```python
from build123d import *

# Parameters (mm, degrees)
SWEEP_THIN1_PROFILE_R   = 15
SWEEP_THIN1_PROFILE_R_2 = 11
SKETCH65_R              = 11
SKETCH65_R_2            = 3
BOSS_EXTRUDE1_DEPTH     = 5
SKETCH66_R              = 11
SKETCH66_R_2            = 3
BOSS_EXTRUDE2_DEPTH     = 5


with BuildPart() as part:
    # Sweep-Thin1: sweep along a path in Sketch1
    with BuildLine(Plane.XY) as sweep_thin1_path:
        ThreePointArc((-45, 0), (-31.819805153, 31.819805153), (0, 45))
    # Sweep-Thin1 profile (on start of the path) → Sweep-Thin1 (sweep)
    with BuildSketch(Plane(origin=(-45, 0, 0), x_dir=(1, 0, 0), z_dir=(0, 1, 0))):
        Circle(SWEEP_THIN1_PROFILE_R)
        Circle(SWEEP_THIN1_PROFILE_R_2, mode=Mode.SUBTRACT)
    sweep(path=sweep_thin1_path.line)

    # Sketch65 → Boss-Extrude1 (add)
    with BuildSketch(Plane(origin=(0, 0, 0), x_dir=(0, 0, -1), z_dir=(1, 0, 0))):
        with BuildLine():
            Line((-5.157087895, 70.566666667), (-15.04150636, 53.944444444))
            ThreePointArc((-15.04150636, 53.944444444), (-17.5, 45), (-15.04150636, 36.055555556))
            Line((-15.04150636, 36.055555556), (-5.157087895, 19.433333333))
            ThreePointArc((-5.157087895, 19.433333333), (0, 16.5), (5.157087895, 19.433333333))
            Line((5.157087895, 19.433333333), (15.04150636, 36.055555556))
            ThreePointArc((15.04150636, 36.055555556), (17.5, 45), (15.04150636, 53.944444444))
            Line((15.04150636, 53.944444444), (5.157087895, 70.566666667))
            ThreePointArc((5.157087895, 70.566666667), (0, 73.5), (-5.157087895, 70.566666667))
        make_face()
        with Locations(Location((0, 45, 0), (0, 0, 90))):
            Circle(SKETCH65_R, mode=Mode.SUBTRACT)
        with Locations(Location((0, 67.5, 0), (0, 0, 90))):
            Circle(SKETCH65_R_2, mode=Mode.SUBTRACT)
        with Locations(Location((0, 22.5, 0), (0, 0, 90))):
            Circle(SKETCH65_R_2, mode=Mode.SUBTRACT)
    extrude(amount=BOSS_EXTRUDE1_DEPTH)

    # Sketch66 → Boss-Extrude2 (add)
    with BuildSketch(Plane.XZ):
        with BuildLine():
            Line((-53.944444444, 15.04150636), (-70.566666667, 5.157087895))
            ThreePointArc((-70.566666667, 5.157087895), (-73.5, 0), (-70.566666667, -5.157087895))
            Line((-70.566666667, -5.157087895), (-53.944444444, -15.04150636))
            ThreePointArc((-53.944444444, -15.04150636), (-45, -17.5), (-36.055555556, -15.04150636))
            Line((-36.055555556, -15.04150636), (-19.433333333, -5.157087895))
            ThreePointArc((-19.433333333, -5.157087895), (-16.5, 0), (-19.433333333, 5.157087895))
            Line((-19.433333333, 5.157087895), (-36.055555556, 15.04150636))
            ThreePointArc((-36.055555556, 15.04150636), (-45, 17.5), (-53.944444444, 15.04150636))
        make_face()
        with Locations(Location((-45, 0, 0), (0, 0, 180))):
            Circle(SKETCH66_R, mode=Mode.SUBTRACT)
        with Locations((-67.5, 0)):
            Circle(SKETCH66_R_2, mode=Mode.SUBTRACT)
        with Locations((-22.5, 0)):
            Circle(SKETCH66_R_2, mode=Mode.SUBTRACT)
    extrude(amount=BOSS_EXTRUDE2_DEPTH)


solid = part.part
```
Work out the finished part from the listing and answer in its coordinate system (mm). A direction names the side the tool comes from. Coordinates: 2 decimals unless noted, no trailing zeros. Write each loop counter-clockwise with the first axis right and the second up, starting at its lowest first coordinate (ties: lowest second). Pieces come first, ordered by that corner, then holes.
Q1. A cutting plane is placed at B-B, the plane z = 6.5. Give the vertices of the cut face in (x, y).
Q2. A cutting plane is placed at D-D, the plane z = 0. State how many separate pieces and enclosed holes the cut face has, then the cut area to 3 significant figures.
Q3. Each of these flat-tipped pins is pushed along its axis until it touches: pin 1 Ø3 at (x, y) = (-58, 5) entering from +Z; pin 2 Ø5 at (y, z) = (55, -3.5) entering from -X; pin 3 Ø10 at (y, z) = (30.5, -11.5) entering from -X. Where does it stop, or does it pass through?
Q4. Which of the six approach directions +Z, -Z, +X, -X, +Y, -Y give full straight-line access (tool end or side, diameter ignored) to faces 4 (the face through (-16.5, -2.5, -0.1)), 5 (the face through (-58, 0, 8)), 6 (the face through (2.465, 55.161, -4.213)), 7 (the face through (-27.63, -2.46, 10.03))?
Q5. A cutting plane is placed at C-C, the plane y = 67.5. Give the vertices of the cut face in (x, z).
Q6. Determine the mould class of faces 1 (the face through (-55.492, -2.465, -3.304)), 2 (the face through (-45.1, -2.5, -17.5)), 3 (the face through (-73.5, -2.5, 0.1)) for opening direction X: released by +X, released by -X, zero draft, split by the parting line, or undercut.
Q7. Find the intervals of material crossed by line 1 (X direction, y = 26, z = 3.5); line 2 (Y direction, x = -24.5, z = -6.5); line 3 (Y direction, x = -14, z = -4), in increasing order.
Q8. A cutting plane is placed at A-A, the plane x = -65.5. Give the vertices of the cut face in (y, z).
Findings below:
1. outline: (-68.31, -5) - (-53.87, -5) - (-53.87, 0) arc R53.87 cw to (0, 53.87) - (5, 53.87) - (5, 68.31) - (0, 68.31) - (0, 58.52) arc R58.52 ccw to (-58.52, 0) - (-68.31, 0) - close; (-36.13, -5) - (-21.69, -5) - (-21.69, 0) - (-31.48, 0) arc R31.48 cw to (0, 31.48) - (0, 21.69) - (5, 21.69) - (5, 36.13) - (0, 36.13) arc R36.13 ccw to (-36.13, 0) - close
2. separate pieces: 6
2. enclosed holes: 0
2. area: 795 mm2
3. pin 1: stops at z = 9.37
3. pin 2: stops at x = -28.32
3. pin 3: stops at x = -51.06
4. face 4: +X, -Y
4. face 5: none
4. face 6: +X
4. face 7: +Z, +X, -Y
5. outline: (0, -6.98) - (5, -6.98) - (5, -3) - (0, -3) - close; (0, 3) - (5, 3) - (5, 6.98) - (0, 6.98) - close
6. face 1: undercut
6. face 2: split by the parting line
6. face 3: released by -X
7. line 1: x = -53.61 to -48.95, -22.79 to -15.78, 0 to 5
7. line 2: y = -5 to 0, 19.77 to 26.55, 47.98 to 53.14
7. line 3: y = 27.15 to 31.81, 53.44 to 57.79
8. outline: (-5, -8.17) - (0, -8.17) - (0, -2.24) - (-5, -2.24) - close; (-5, 2.24) - (0, 2.24) - (0, 8.17) - (-5, 8.17) - close
